Build history of the part. All positions in model axes, mm. Give positions to 0.01 mm unless a question says otherwise; leave off trailing zeros. Write each loop counter-clockwise with the first axis right and the second up, starting at its lowest first coordinate (ties: lowest second). Pieces come first, ordered by that corner, then holes. Notation, with made-up numbers: (-20, 64) - (-15, 64) arc R26 ccw to (-15, 96) - close; hole circle Ø5 at (71, 85). An arc over 180 degrees is marked (long way). Use one line per item in the form item = value. Start each with the question number.
from build123d import *

# Parameters (mm, degrees)
SKETCH1_W           = 152.4
SKETCH1_H           = 152.4
BOSS_EXTRUDE1_DEPTH = 3.175
BOSS_EXTRUDE2_DEPTH = 0.635
SKETCH3_W           = 2.54
SKETCH3_H           = 2.54
CUT_EXTRUDE1_DEPTH  = 4.175


with BuildPart() as part:
    # Sketch1 → Boss-Extrude1 (new body)
    with BuildSketch(Plane(origin=(0, 0, 0), x_dir=(1, 0, 0), z_dir=(0, 1, 0))):
        with Locations((76.2, 76.2)):
            Rectangle(SKETCH1_W, SKETCH1_H)
    extrude(amount=BOSS_EXTRUDE1_DEPTH)

    # Sketch2 → Boss-Extrude2 (add)
    with BuildSketch(Plane(origin=(0, 3.175, 0), x_dir=(1, 0, 0), z_dir=(0, 1, 0))):
        Polygon((0, 152.4), (-2.54, 152.4), (-2.54, -2.54), (152.4, -2.54), (152.4, 0), (0, 0), align=None)
    extrude(amount=-BOSS_EXTRUDE2_DEPTH)

    # Sketch3 → Cut-Extrude1 (cut, through all)
    with BuildSketch(Plane(origin=(0, 3.175, 0), x_dir=(1, 0, 0), z_dir=(0, 1, 0))):
        with Locations((-1.27, -1.27)):
            Rectangle(SKETCH3_W, SKETCH3_H)
    extrude(amount=-CUT_EXTRUDE1_DEPTH, mode=Mode.SUBTRACT)


solid = part.part
(1) Pin check, flat tips, straight feed: pin 1 Ø6 at (x, z) = (91, -14) entering from -Y; pin 2 Ø0.8 at (x, z) = (-1.5, -55) entering from -Y; pin 3 Ø1.3 at (y, z) = (1, -39.5) entering from -X; pin 4 Ø0.8 at (x, y) = (61.5, 1) entering from +Z. Stop position of each tip, or through.
(2) Cut at A-A, the plane y = 1.35. Give the cut face in (x, z), then the cut area to 3 significant figures.
(3) Wall check: line 1 (Z direction, x = 55, y = 1.3); line 2 (X direction, y = 2.3, z = -126.5). Give the ranges that are in metal, low to high. Write a range as from..to.
Solution:
q1.pin_1 = 0
q1.pin_2 = 2.54
q1.pin_3 = 0
q1.pin_4 = 0
q2.outline = (0, -152.4) - (152.4, -152.4) - (152.4, 0) - (0, 0) - close
q2.area = 23,200 mm2
q3.line_1 = -152.4..0
q3.line_2 = 0..152.4
